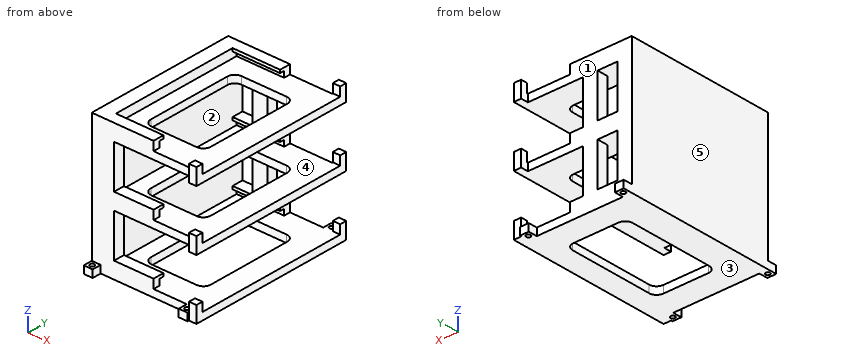
```python
from build123d import *

# Parameters (mm, degrees)
BOSS_EXTRUDE1_DEPTH     = 5
SKETCH4_W               = 5
SKETCH4_H               = 4.5
BOSS_EXTRUDE2_DEPTH     = 6
SKETCH5_W               = 3
SKETCH5_H               = 2
BOSS_EXTRUDE3_DEPTH     = 32
SKETCH6_W               = 6
SKETCH6_H               = 6
BOSS_EXTRUDE4_DEPTH     = 5
BOSS_EXTRUDE4_2_DEPTH   = 5
BOSS_EXTRUDE4_3_DEPTH   = 5
BOSS_EXTRUDE4_4_DEPTH   = 5
SKETCH7_R               = 1.5
CUT_EXTRUDE1_DEPTH      = 6
LPATTERN1_COUNT         = 3
LPATTERN1_PITCH         = 40
SKETCH8_W               = 10
SKETCH8_H               = 7.4
BOSS_EXTRUDE5_DEPTH     = 29
SKETCH9_W               = 10
SKETCH9_H               = 7.4
BOSS_EXTRUDE6_DEPTH     = 29
CUT_EXTRUDE2_DEPTH      = 7
CUT_EXTRUDE2_DEPTH_BACK = 86


with BuildPart() as part:
    # Sketch1 → Boss-Extrude1 (new body)
    with BuildSketch(Plane(origin=(0, 0, 0), x_dir=(0, 1, 0), z_dir=(0, 0, 1))):
        Polygon((-51, 5), (-51, 75), (51, 75), (51, 5), (56, 5), (56, 0), (-56, 0), (-56, 5), align=None)
    extrude(amount=BOSS_EXTRUDE1_DEPTH)

    # Sketch4 → Boss-Extrude2 (add)
    with BuildSketch(Plane.XY.offset(5)):
        Polygon((-75, 51), (-75, -51), (-33.4, -51), (-33.4, -46.6), (-65.4, -46.6), (-65.4, 46.6), (-33.4, 46.6), (-33.4, 51), align=None)
        with Locations((-2.5, 53.75)):
            Rectangle(SKETCH4_W, SKETCH4_H)
        with Locations((-2.5, -53.75)):
            Rectangle(SKETCH4_W, SKETCH4_H)
    extrude(amount=BOSS_EXTRUDE2_DEPTH)

    # Sketch5 → Boss-Extrude3 (add)
    with BuildSketch(Plane.YZ.offset(-65.4)):
        with Locations((-45.1, 10)):
            Rectangle(SKETCH5_W, SKETCH5_H)
        with Locations((45.1, 10)):
            Rectangle(SKETCH5_W, SKETCH5_H)
    extrude(amount=BOSS_EXTRUDE3_DEPTH)


with BuildPart() as body_2:
    # Sketch6 → Boss-Extrude4 (new body)
    with BuildSketch(Plane(origin=(0, 0, 0), x_dir=(1, 0, 0), z_dir=(0, 0, -1))):
        with Locations((-8, 54)):
            Rectangle(SKETCH6_W, SKETCH6_H)
    extrude(amount=-BOSS_EXTRUDE4_DEPTH)


with BuildPart() as body_3:
    # Sketch6 → Boss-Extrude4 2 (new body)
    with BuildSketch(Plane(origin=(0, 0, 0), x_dir=(1, 0, 0), z_dir=(0, 0, -1))):
        with Locations((-72, 54)):
            Rectangle(SKETCH6_W, SKETCH6_H)
    extrude(amount=-BOSS_EXTRUDE4_2_DEPTH)


with BuildPart() as body_4:
    # Sketch6 → Boss-Extrude4 3 (new body)
    with BuildSketch(Plane(origin=(0, 0, 0), x_dir=(1, 0, 0), z_dir=(0, 0, -1))):
        with Locations((-8, -54)):
            Rectangle(SKETCH6_W, SKETCH6_H)
    extrude(amount=-BOSS_EXTRUDE4_3_DEPTH)


with BuildPart() as body_5:
    # Sketch6 → Boss-Extrude4 4 (new body)
    with BuildSketch(Plane(origin=(0, 0, 0), x_dir=(1, 0, 0), z_dir=(0, 0, -1))):
        with Locations((-72, -54)):
            Rectangle(SKETCH6_W, SKETCH6_H)
    extrude(amount=-BOSS_EXTRUDE4_4_DEPTH)


with BuildPart() as cut_extrude1_tool:
    # Sketch7 → Cut-Extrude1 (new body, through all)
    with BuildSketch(Plane.XY.offset(5)):
        with Locations((-8, -54)):
            Circle(SKETCH7_R)
        with Locations((-72, -54)):
            Circle(SKETCH7_R)
        with Locations((-8, 54)):
            Circle(SKETCH7_R)
        with Locations((-72, 54)):
            Circle(SKETCH7_R)
    extrude(amount=-CUT_EXTRUDE1_DEPTH)


with BuildPart() as body_2_1:
    add(body_2.part)

    # Cut-Extrude1: cut by cut_extrude1_tool
    add(cut_extrude1_tool.part, mode=Mode.SUBTRACT)


with BuildPart() as body_3_1:
    add(body_3.part)

    # Cut-Extrude1: cut by cut_extrude1_tool
    add(cut_extrude1_tool.part, mode=Mode.SUBTRACT)


with BuildPart() as body_4_1:
    add(body_4.part)

    # Cut-Extrude1: cut by cut_extrude1_tool
    add(cut_extrude1_tool.part, mode=Mode.SUBTRACT)


with BuildPart() as body_5_1:
    add(body_5.part)

    # Cut-Extrude1: cut by cut_extrude1_tool
    add(cut_extrude1_tool.part, mode=Mode.SUBTRACT)


with BuildPart() as lpattern1_1:
    # LPattern1: pattern copy
    add(part.part.moved(Location(Vector(0, 0, 1) * (1 * LPATTERN1_PITCH))))



with BuildPart() as lpattern1_2:
    # LPattern1: pattern copy
    add(part.part.moved(Location(Vector(0, 0, 1) * (2 * LPATTERN1_PITCH))))


with BuildPart() as part_1:
    add(part.part)

    # Sketch8 → Boss-Extrude5 (add)
    with BuildSketch(Plane.XY.offset(11)):
        with Locations((-47, 47.3)):
            Rectangle(SKETCH8_W, SKETCH8_H)
        Polygon((-65.4, 51), (-65.4, -43.6), (-60, -43.6), (-60, -51), (-75, -51), (-75, 51), align=None)
    extrude(amount=BOSS_EXTRUDE5_DEPTH)


with BuildPart() as lpattern1_1_1:
    add(lpattern1_1.part)

    add(lpattern1_2.part)  # Boss-Extrude6 merges LPattern1_2
    # Sketch9 → Boss-Extrude6 (add)
    with BuildSketch(Plane.XY.offset(51)):
        with Locations((-47, 47.3)):
            Rectangle(SKETCH9_W, SKETCH9_H)
        Polygon((-65.4, 51), (-65.4, -43.6), (-60, -43.6), (-60, -51), (-75, -51), (-75, 51), align=None)
    extrude(amount=BOSS_EXTRUDE6_DEPTH)

    # Combine1: union part, body 3, body 2, body 5, body 4
    add(part_1.part)
    add(body_3_1.part)
    add(body_2_1.part)
    add(body_5_1.part)
    add(body_4_1.part)

    # Sketch10 → Cut-Extrude2 (cut, two sides)
    with BuildSketch(Plane.XY.offset(85)) as cut_extrude2_sk:
        with BuildLine():
            Line((-50.4, 33.6), (-20, 33.6))
            ThreePointArc((-20, 33.6), (-16.464466094, 32.135533906), (-15, 28.6))
            Line((-15, 28.6), (-15, -28.6))
            ThreePointArc((-15, -28.6), (-16.464466094, -32.135533906), (-20, -33.6))
            Line((-20, -33.6), (-50.4, -33.6))
            ThreePointArc((-50.4, -33.6), (-53.935533906, -32.135533906), (-55.4, -28.6))
            Line((-55.4, -28.6), (-55.4, 28.6))
            ThreePointArc((-55.4, 28.6), (-53.935533906, 32.135533906), (-50.4, 33.6))
        make_face()
    extrude(amount=CUT_EXTRUDE2_DEPTH, mode=Mode.SUBTRACT)
    extrude(cut_extrude2_sk.sketch, amount=-CUT_EXTRUDE2_DEPTH_BACK, mode=Mode.SUBTRACT)


solid = lpattern1_1_1.part
```
Design review of the part built by this model. Coordinates are the model's own, in mm. Face numbers are marked on the shaded views. A direction names the side the tool comes from. Coordinates: 2 decimals unless noted, no trailing zeros. Loops run counter-clockwise (first coordinate to the right, second up) from the corner with the lowest first, then second, coordinate; pieces in that order, holes last.
Q1. We need section C-C on y = 16. State the section outline as (x, z) points.
Reported:
outline: (-75, 0) - (-55.4, 0) - (-55.4, 5) - (-65.4, 5) - (-65.4, 40) - (-55.4, 40) - (-55.4, 45) - (-65.4, 45) - (-65.4, 80) - (-55.4, 80) - (-55.4, 85) - (-65.4, 85) - (-65.4, 91) - (-75, 91) - close; (-15, 0) - (0, 0) - (0, 5) - (-15, 5) - close; (-15, 40) - (0, 40) - (0, 45) - (-15, 45) - close; (-15, 80) - (0, 80) - (0, 85) - (-15, 85) - close
Q2. Tool access review of the marked faces 4 and 5: name each direction out of +Z, -Z, +X, -X, +Y, -Y from which nothing blocks a thin tool from reaching the whole face with its end or side.
Reported:
face 4: +X
face 5: +Z, -Z, -X, +Y, -Y
Q3. To check wall thickness, follow line 1 (Z direction, x = -18, y = 37); line 2 (Y direction, x = -8, z = 2); line 3 (Z direction, x = -35.5, y = -44). State the ranges of each line that lie inside material, in increasing order.
Reported:
line 1: z = 0 to 5, 40 to 45, 80 to 85
line 2: y = -57 to -55.5, -52.5 to 52.5, 55.5 to 57
line 3: z = 0 to 5, 9 to 11, 40 to 45, 49 to 51, 80 to 85, 89 to 91
Q4. We need section A-A on z = 22.5. State the section outline as (x, y) points, and give its area (3 significant figures).
Reported:
outline: (-75, -51) - (-60, -51) - (-60, -43.6) - (-65.4, -43.6) - (-65.4, 51) - (-75, 51) - close; (-52, 43.6) - (-42, 43.6) - (-42, 51) - (-52, 51) - close
area: 1,090 mm2
Q5. The part is to be moulded in two halves that separate along Z. For the marked faces 1, 2 and 3, say which applies: +Z half, -Z half, draft (parallel to the pull), parting line (faces both ways), or undercut.
Reported:
face 1: draft
face 2: undercut
face 3: -Z half
Q6. For pin 1 (2.5 mm diameter, centred on x = -3, z = 89.5, fed in from -Y); pin 2 (1.8 mm diameter, centred on x = -71.5, y = -55.5, fed in from +Z); pin 3 (1 mm diameter, centred on y = 30.5, z = 33, fed in from +X), all flat-tipped, find the tip position at first contact; note any pin that passes through.
Reported:
pin 1: stops at y = -56
pin 2: stops at z = 5
pin 3: stops at x = -65.4
Q7. We need section D-D on x = -72. State the section outline as (y, z) points, and give its area (3 significant figures).
Reported:
outline: (-57, 0) - (-55.5, 0) - (-55.5, 5) - (-57, 5) - close; (-52.5, 0) - (52.5, 0) - (52.5, 5) - (51, 5) - (51, 91) - (-51, 91) - (-51, 5) - (-52.5, 5) - close; (55.5, 0) - (57, 0) - (57, 5) - (55.5, 5) - close
area: 9,310 mm2
Q8. We need section B-B on x = -8. State the section outline as (y, z) points, and give its area (3 significant figures).
Reported:
outline: (-57, 0) - (-55.5, 0) - (-55.5, 5) - (-57, 5) - close; (-52.5, 0) - (52.5, 0) - (52.5, 5) - (-52.5, 5) - close; (-51, 40) - (51, 40) - (51, 45) - (-51, 45) - close; (-51, 80) - (51, 80) - (51, 85) - (-51, 85) - close; (55.5, 0) - (57, 0) - (57, 5) - (55.5, 5) - close
area: 1,560 mm2
